```python
from build123d import *

# Parameters (mm, degrees)
F0_W   = 2.54
F0_H   = 2.54
F0_H_2 = 76.962


with BuildPart() as f1:
    # F0 (on Front) → F1 (revolve)
    with BuildSketch(Plane.XZ):
        Polygon((-26.96, 33.528), (0, 33.528), (26.96, 33.528), (26.96, 36.068), (0, 36.068), (-26.96, 36.068), align=None)
        with Locations((28.23, 34.798)):
            Rectangle(F0_W, F0_H)
        with Locations((-28.23, 34.798)):
            Rectangle(F0_W, F0_H)
        with Locations((28.23, 74.549)):
            Rectangle(F0_W, F0_H_2)
        with Locations((-28.23, 74.549)):
            Rectangle(F0_W, F0_H_2)
    revolve(axis=Axis((13.856179, 0, 0), (1, 0, 0)))


solid = f1.part
```
Design review of the part built by this model. Coordinates are the model's own, in mm. A direction names the side the tool comes from. Coordinates: 2 decimals unless noted, no trailing zeros. Loops run counter-clockwise (first coordinate to the right, second up) from the corner with the lowest first, then second, coordinate; pieces in that order, holes last. Notation, with made-up numbers: (79.5, 75) -> (103.5, 75) arc R15 cw to (103.5, 87) -> close; hole circle Ø1 at (31, 84.5). An arc over 180 degrees is marked (long way). Answer as a JSON object with one key per item and string values.
Q1. Clearance check with flat-ended pins moving along their axes: pin 1 Ø12 at (x, y) = (-1.5, 23.5) entering from -Z; pin 2 Ø1.5 at (x, z) = (-18.5, -26.5) entering from +Y; pin 3 Ø4 at (x, z) = (-1.5, -12) entering from -Y. State where each tip first meets the part, or that it passes through.
Answer block:
{"pin 1": "stops at z = -31.54", "pin 2": "stops at y = 25.26", "pin 3": "stops at y = -34.65"}
Q2. Tool access review of faces 5 (the flat face through (-26.96, -27, 27)), 6 (the cylindrical face through (28.248, 68.777, -89.697)): name each direction out of +Z, -Z, +X, -X, +Y, -Y from which nothing blocks a thin tool from reaching the whole face with its end or side.
Answer block:
{"face 5": "none", "face 6": "+X, -X"}
Q3. The part is to be moulded in two halves that separate along X. For faces 1 (the cylindrical face through (0, -10, 32)), 2 (the flat face through (26.96, -27, 27)), 3 (the flat face through (-29.5, -27, 24)), 4 (the cylindrical face through (-0.38, 35.21, -7.82)), say which applies: +X half, -X half, draft (parallel to the pull), parting line (faces both ways), or undercut.
Answer block:
{"face 1": "draft", "face 2": "undercut", "face 3": "-X half", "face 4": "undercut"}
Q4. Take a section at A-A on z = 0. Give the boundary of the cut face in (x, y), plus the area to 3 significant figures.
Answer block:
{"outline": "(-29.5, -113.03) -> (-26.96, -113.03) -> (-26.96, -36.07) -> (26.96, -36.07) -> (26.96, -113.03) -> (29.5, -113.03) -> (29.5, -33.53) -> (-29.5, -33.53) -> close; (-29.5, 33.53) -> (29.5, 33.53) -> (29.5, 113.03) -> (26.96, 113.03) -> (26.96, 36.07) -> (-26.96, 36.07) -> (-26.96, 113.03) -> (-29.5, 113.03) -> close", "area": "1,080 mm^2"}
Q5. Take a section at C-C on x = 8. Give the boundary of the cut face in (y, z), plus the area to 3 significant figures.
Answer block:
{"outline": "circle Ø72.14 at (0, 0); hole circle Ø67.06 at (0, 0)", "area": "555 mm^2"}
Q6. Take a section at D-D on y = -43.5. Give the boundary of the cut face in (x, z).
Answer block:
{"outline": "(-29.5, -104.32) -> (-26.96, -104.32) -> (-26.96, 104.32) -> (-29.5, 104.32) -> close; (26.96, -104.32) -> (29.5, -104.32) -> (29.5, 104.32) -> (26.96, 104.32) -> close"}
Q7. To check wall thickness, follow L1, parallel to Z at x = 3.5, y = 0; L2, parallel to X at y = -15, z = -34. State the ranges of each line that lie inside material, in increasing order.
Answer block:
{"L1": "z = -36.07 to -33.53, 33.53 to 36.07", "L2": "x = -29.5 to -26.96, 26.96 to 29.5"}
